Study the drawing (mm; zero at the part's minimum x, y, z) and answer. A direction names the side the tool comes from. Coordinates: 2 decimals unless noted, no trailing zeros. Write each loop counter-clockwise with the first axis right and the second up, starting at its lowest first coordinate (ties: lowest second). Pieces come first, ordered by that corner, then holes. Notation, with made-up numbers: (48.5, 58) - (101.5, 58) arc R22 cw to (101.5, 67) - close; hole circle Ø6 at (-3.5, 15). An arc over 180 degrees is marked (long way). One line per item, written item: value.
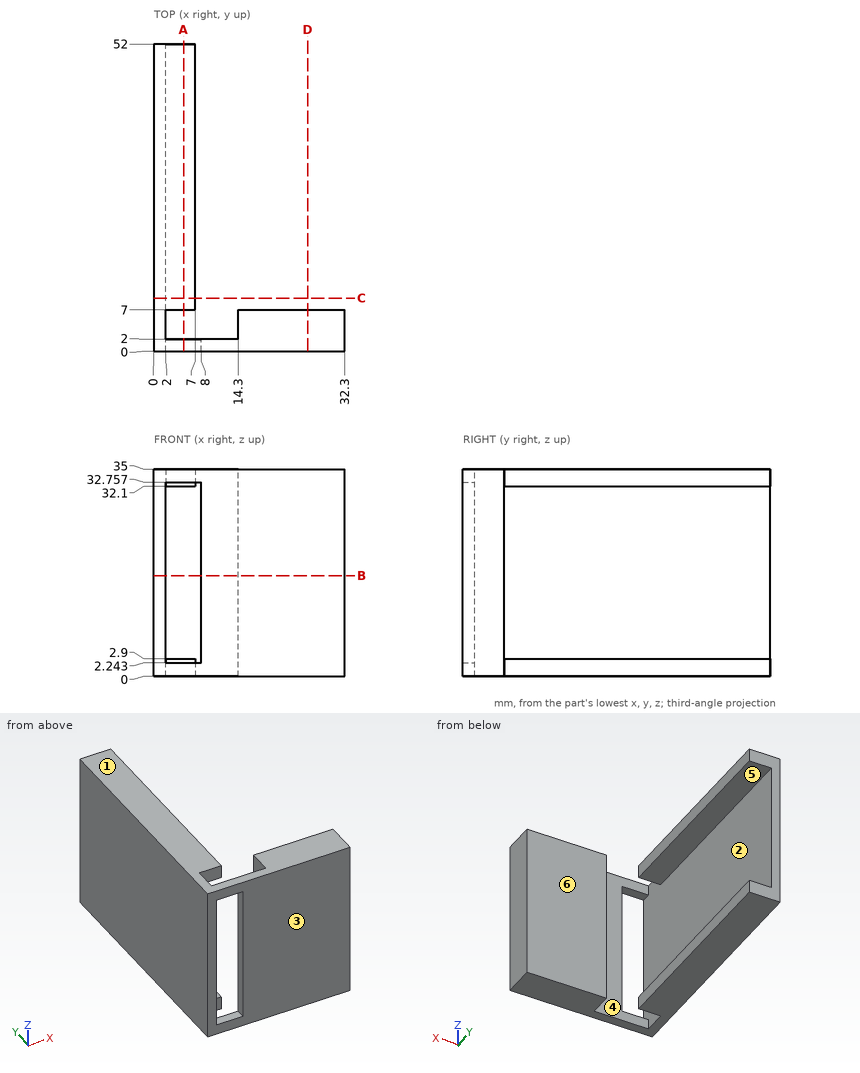
Item 1: Section B-B, the plane z = 17 is taken. Determine the outline of the cut face in (x, y).
Evaluation:
outline: (0, 0) - (2, 0) - (2, 52) - (0, 52) - close; (8, 0) - (32.3, 0) - (32.3, 7) - (14.3, 7) - (14.3, 2) - (8, 2) - close
Item 2: Consider probe 1 along Y at (x, z) = (6.5, 33); probe 2 along Z at (x, y) = (3.5, 26); probe 3 along X at (y, z) = (6.5, 17.5). Determine where each line is inside the solid, lowest interval first.
Evaluation:
probe 1: y = 0 to 2, 7 to 52
probe 2: z = 0 to 2.9, 32.1 to 35
probe 3: x = 0 to 2, 14.3 to 32.3
Item 3: Section A-A, the plane x = 5 is taken. Determine the outline of the cut face in (y, z), then the cut area to 3 significant figures.
Evaluation:
outline: (0, 0) - (2, 0) - (2, 2.24) - (0, 2.24) - close; (0, 32.76) - (2, 32.76) - (2, 35) - (0, 35) - close; (7, 0) - (52, 0) - (52, 2.9) - (7, 2.9) - close; (7, 32.1) - (52, 32.1) - (52, 35) - (7, 35) - close
area: 270 mm2
Item 4: Which of the six approach directions +Z, -Z, +X, -X, +Y, -Y give full straight-line access (tool end or side, diameter ignored) to the marked faces 4, 5 and 6?
Evaluation:
face 4: +Z, -Z
face 5: +X, +Y, -Y
face 6: +Z, -Z, +X, +Y
Item 5: Section D-D, the plane x = 26 is taken. Determine the outline of the cut face in (y, z).
Evaluation:
outline: (0, 0) - (7, 0) - (7, 35) - (0, 35) - close
Item 6: Section C-C, the plane y = 9 is taken. Determine the outline of the cut face in (x, z), then the cut area to 3 significant figures.
Evaluation:
outline: (0, 0) - (7, 0) - (7, 2.9) - (2, 2.9) - (2, 32.1) - (7, 32.1) - (7, 35) - (0, 35) - close
area: 99.0 mm2
Item 7: Determine the mould class of the marked faces 1, 2 and 3 for opening direction Z: +Z half, -Z half, draft (parallel to the pull), parting line (faces both ways), or undercut.
Evaluation:
face 1: +Z half
face 2: undercut
face 3: draft
Item 8: Given pin 1 (3 mm diameter, centred on y = 38, z = 33.5, fed in from +X); pin 2 (6 mm diameter, centred on x = 7.5, z = 11.5, fed in from +Y); pin 3 (4 mm diameter, centred on y = 37.5, z = 28, fed in from +X), each flat-ended and moving along its own axis, determine where each tip first touches the part or whether it passes through.
Evaluation:
pin 1: stops at x = 7
pin 2: stops at y = 2
pin 3: stops at x = 2
